The figure shows three views and two pictorial views of one solid part (mm, origin at its lowest corner). Answer the questions. Round coordinates to 2 decimals unless told otherwise and drop trailing zeros. Order: outer loops, then holes, each group sorted by start corner. A loop starts at its lowest first (then second) coordinate and runs counter-clockwise, first axis right, second up. Notation, with made-up numbers: (-2.75, 34.5) - (39.25, 34.5) arc R38 ccw to (39.25, 72.5) - close; hole circle Ø6 at (56, 61). An arc over 180 degrees is marked (long way). Answer in a Markdown table with one row per item.
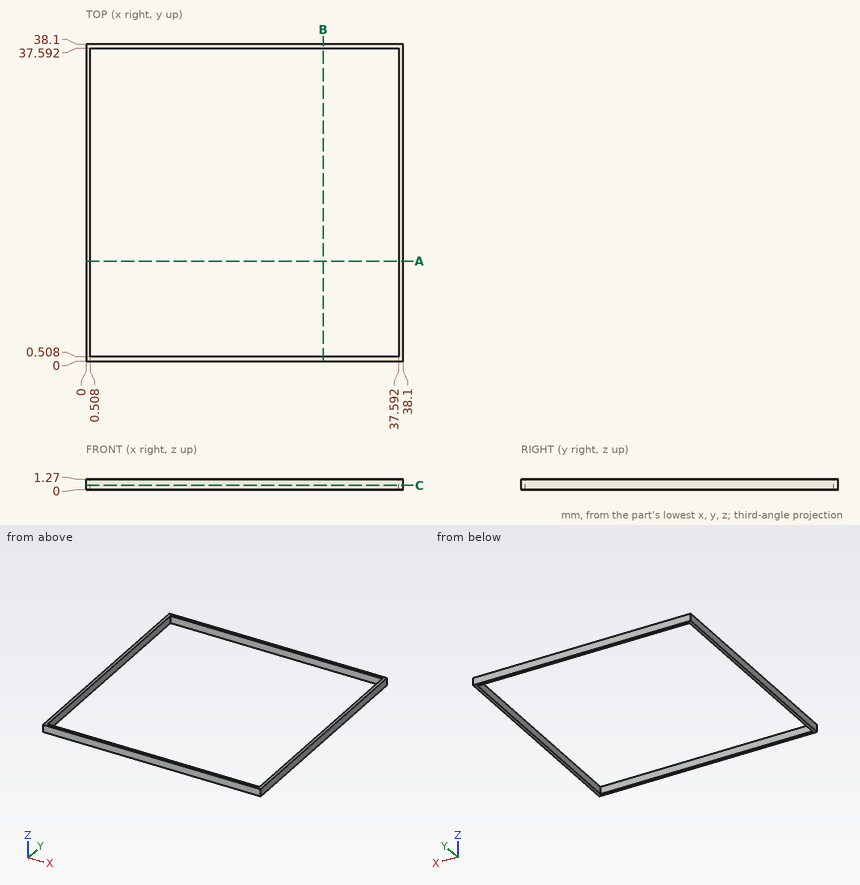
1) Find section A-A, the plane y = 12. Give the vertices of the cut face in (x, z).
Filled in:
| item | result |
|---|---|
| outline | (0, 0) - (0.51, 0) - (0.51, 1.27) - (0, 1.27) - close; (37.59, 0) - (38.1, 0) - (38.1, 1.27) - (37.59, 1.27) - close |
2) Find the intervals of material crossed by probe 1 along X at (y, z) = (12.5, 0.3), in increasing order. Write a range as from..to.
Filled in:
| item | result |
|---|---|
| probe 1 | x = 0..0.51, 37.59..38.1 |
3) Find section C-C, the plane z = 0.5. Give the vertices of the cut face in (x, y).
Filled in:
| item | result |
|---|---|
| outline | (0, 0) - (38.1, 0) - (38.1, 38.1) - (0, 38.1) - close; hole (0.51, 0.51) - (37.59, 0.51) - (37.59, 37.59) - (0.51, 37.59) - close |
